Here's how the part is built. I have some questions about the finished solid (model axes, mm). Face numbers are marked on the shaded views. A direction names the side the tool comes from. Give positions to 0.01 mm unless a question says otherwise; leave off trailing zeros. Loops run counter-clockwise (first coordinate to the right, second up) from the corner with the lowest first, then second, coordinate; pieces in that order, holes last.
Q1. Suppose I cut it at A-A (x = 4). List the corners of the cut face in (y, z) for me, and give its area (3 significant figures).
Q2. Thinking about a two-plate mould opening in X: for the marked faces 1, 2, 3 and 4, which applies, pulls with the +X half, pulls with the -X half, needs draft (parallel to the pull), parting line crosses it, or undercut?
Q3. Suppose I cut it at D-D (z = 107.5). List the corners of the cut face in (x, y) for me.
Q4. Suppose I cut it at C-C (z = 150). List the corners of the cut face in (x, y) for me.
Q5. For the marked faces 5 and 6, which set-ups out of +Z, -Z, +X, -X, +Y, -Y let a thin tool reach every point of the face, with its end or its side?
Q6. Suppose I cut it at B-B (y = 8.5). List the corners of the cut face in (x, z) for me, and give its area (3 significant figures).
Q7. I'm going to push flat-ended pins straight in: P1, Ø1.5, axis at x = -31, z = 131.5, coming from the -Y side; P2, Ø1.5, axis at x = -18.5, y = -3, coming from the +Z side; P3, Ø18, axis at x = -15.5, z = 11, coming from the +Y side. Where does each tip first touch, or does it pass through?
Q8. I need wall thicknesses on probe 1 along X at (y, z) = (15.5, 65); probe 2 along Y at (x, z) = (43, 60); probe 3 along Y at (x, z) = (33.5, 79.5). Which ranges of each line are inside material? Lowest first, please.
```python
from build123d import *

# Parameters (mm, degrees)
SKETCH_1_W          = 5
SKETCH_1_H          = 10
EXTRUDE_1_DEPTH     = 240
SKETCH_3_R          = 2.1
SKETCH_3_R_2        = 5.5
CUT_EXTRUDE_1_DEPTH = 90
CUT_EXTRUDE_2_DEPTH = 80
SKETCH_8_W          = 24
SKETCH_8_H          = 5
CUT_EXTRUDE_3_DEPTH = 80


# Read off the part's stored shape, not the designer's step: 切除-拉伸2
with BuildPart() as part:
    # 草图1 → 凸台-拉伸1 (new body)
    with BuildSketch(Plane.XY):
        Polygon((0, -5), (0, 0), (-40, 0), (-40, 25), (-45, 25), (-45, -5), (-40, -5), align=None)
        Polygon((40, 25), (40, 0), (0, 0), (0, -5), (40, -5), (45, -5), (45, 25), align=None)
        with Locations((-42.5, -10)):
            Rectangle(SKETCH_1_W, SKETCH_1_H)
        with Locations((42.5, -10)):
            Rectangle(SKETCH_1_W, SKETCH_1_H)
    extrude(amount=EXTRUDE_1_DEPTH)

    # 草图3 → 切除-拉伸1 (cut, symmetric)
    with BuildSketch(Plane.ZY.offset(-40)):
        Polygon((240, -15), (240, -5), (230.53341221, -9.845037717), (214.283999291, -15), align=None)
        with Locations(Location((231.464466094, -6.464466094, 0), (0, 0, 90))):
            Circle(SKETCH_3_R)
        with Locations(Location((30, -6, 0), (0, 0, 90))):
            Circle(SKETCH_3_R_2)
        with Locations(Location((60, -6, 0), (0, 0, 90))):
            Circle(SKETCH_3_R_2)
        with Locations(Location((90, -6, 0), (0, 0, 90))):
            Circle(SKETCH_3_R_2)
        with Locations(Location((120, -6, 0), (0, 0, 90))):
            Circle(SKETCH_3_R_2)
        with Locations(Location((150, -6, 0), (0, 0, 90))):
            Circle(SKETCH_3_R_2)
        with Locations(Location((180, -6, 0), (0, 0, 90))):
            Circle(SKETCH_3_R_2)
        with Locations(Location((219.464466094, -6.464466094, 0), (0, 0, 90))):
            Circle(SKETCH_3_R)
    extrude(amount=CUT_EXTRUDE_1_DEPTH, both=True, mode=Mode.SUBTRACT)

    # 切除-拉伸2 outline → 切除-拉伸2 (cut)
    with BuildSketch(Plane(origin=(-40, 0, 0), x_dir=(0, 0, -1), z_dir=(1, 0, 0))):
        with BuildLine():
            Line((-82.5, -5), (-82.5, 0))
            Line((-82.5, 0), (-97.5, 0))
            Line((-97.5, 0), (-97.5, -5))
            Line((-97.5, -5), (-95.408326913, -5))
            ThreePointArc((-95.408326913, -5), (-90, -0.5), (-84.591673087, -5))
            Line((-84.591673087, -5), (-82.5, -5))
        make_face()
        with BuildLine():
            Line((-52.5, 0), (-67.5, 0))
            Line((-67.5, 0), (-67.5, -5))
            Line((-67.5, -5), (-65.408326913, -5))
            ThreePointArc((-65.408326913, -5), (-60, -0.5), (-54.591673087, -5))
            Line((-54.591673087, -5), (-52.5, -5))
            Line((-52.5, -5), (-52.5, 0))
        make_face()
        with BuildLine():
            Line((-112.5, -5), (-112.5, 0))
            Line((-112.5, 0), (-127.5, 0))
            Line((-127.5, 0), (-127.5, -5))
            Line((-127.5, -5), (-125.408326913, -5))
            ThreePointArc((-125.408326913, -5), (-120, -0.5), (-114.591673087, -5))
            Line((-114.591673087, -5), (-112.5, -5))
        make_face()
        with BuildLine():
            Line((-22.5, 0), (-37.5, 0))
            Line((-37.5, 0), (-37.5, -5))
            Line((-37.5, -5), (-35.408326913, -5))
            ThreePointArc((-35.408326913, -5), (-30, -0.5), (-24.591673087, -5))
            Line((-24.591673087, -5), (-22.5, -5))
            Line((-22.5, -5), (-22.5, 0))
        make_face()
        with BuildLine():
            Line((-142.5, -5), (-142.5, 0))
            Line((-142.5, 0), (-157.5, 0))
            Line((-157.5, 0), (-157.5, -5))
            Line((-157.5, -5), (-155.408326913, -5))
            ThreePointArc((-155.408326913, -5), (-150, -0.5), (-144.591673087, -5))
            Line((-144.591673087, -5), (-142.5, -5))
        make_face()
        with BuildLine():
            Line((-172.5, -5), (-172.5, 0))
            Line((-172.5, 0), (-187.5, 0))
            Line((-187.5, 0), (-187.5, -5))
            Line((-187.5, -5), (-185.408326913, -5))
            ThreePointArc((-185.408326913, -5), (-180, -0.5), (-174.591673087, -5))
            Line((-174.591673087, -5), (-172.5, -5))
        make_face()
    extrude(amount=CUT_EXTRUDE_2_DEPTH, mode=Mode.SUBTRACT)

    # 草图8 → 切除-拉伸3 (cut)
    with BuildSketch(Plane(origin=(-40, 0, 0), x_dir=(0, 0, -1), z_dir=(1, 0, 0))):
        with Locations((-228, -2.5)):
            Rectangle(SKETCH_8_W, SKETCH_8_H)
    extrude(amount=CUT_EXTRUDE_3_DEPTH, mode=Mode.SUBTRACT)


solid = part.part
```
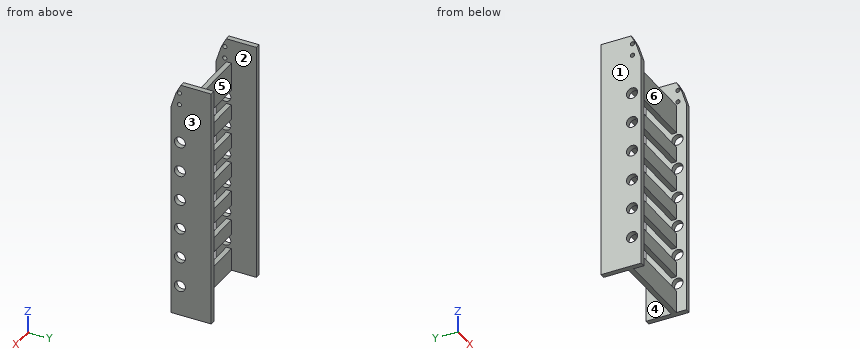
Solutions:
1. outline: (-5, 0) - (0, 0) - (0, 22.5) - (-5, 22.5) - close; (-5, 37.5) - (0, 37.5) - (0, 52.5) - (-5, 52.5) - close; (-5, 67.5) - (0, 67.5) - (0, 82.5) - (-5, 82.5) - close; (-5, 97.5) - (0, 97.5) - (0, 112.5) - (-5, 112.5) - close; (-5, 127.5) - (0, 127.5) - (0, 142.5) - (-5, 142.5) - close; (-5, 157.5) - (0, 157.5) - (0, 172.5) - (-5, 172.5) - close; (-5, 187.5) - (0, 187.5) - (0, 216) - (-5, 216) - close
1. area: 630 mm2
2. face 1: pulls with the -X half
2. face 2: undercut
2. face 3: pulls with the +X half
2. face 4: undercut
3. outline: (-45, -15) - (-40, -15) - (-40, -5) - (40, -5) - (40, -15) - (45, -15) - (45, 25) - (40, 25) - (40, 0) - (-40, 0) - (-40, 25) - (-45, 25) - close
4. outline: (-45, -15) - (-40, -15) - (-40, -11.5) - (-45, -11.5) - close; (-45, -0.5) - (-40, -0.5) - (-40, 25) - (-45, 25) - close; (40, -15) - (45, -15) - (45, -11.5) - (40, -11.5) - close; (40, -0.5) - (45, -0.5) - (45, 25) - (40, 25) - close
5. face 5: +Z, -Z, +Y
5. face 6: +Z, -Z, -Y
6. outline: (-45, 0) - (-40, 0) - (-40, 240) - (-45, 240) - close; (40, 0) - (45, 0) - (45, 240) - (40, 240) - close
6. area: 2,400 mm2
7. P1: stops at y = -5
7. P2: stops at z = 216
7. P3: stops at y = 0
8. probe 1: x = -45 to -40, 40 to 45
8. probe 2: y = -15 to -11.5, -0.5 to 25
8. probe 3: y = -5 to 0
